Source: CAD feature listing. Evaluate the final solid. Frame: model axes, mm. Face numbers are marked on the shaded views. A direction names the side the tool comes from. Round coordinates to 2 decimals unless told otherwise and drop trailing zeros. Order: outer loops, then holes, each group sorted by start corner. A loop starts at its lowest first (then second) coordinate and runs counter-clockwise, first axis right, second up. Notation, with made-up numbers: (-26, 17) - (13, 17) arc R17 ccw to (13, 42) - close; hole circle Ø6 at (60, 69.5). An arc over 180 degrees is marked (long way). Return JSON: item names as keys, results as strings. Group by question number.
1) Section A-A, the plane z = -36.5. Return loops of the section in (x, y).
2) Ray query, line 1 (Y direction, x = 21, z = 45); line 2 (Y direction, x = 3, z = -17); line 3 (Z direction, x = 15, y = 56.5). Return the intervals inside material, ascending. Write a range as from..to.
3) Mould query, pull axis X, two halves, no side actions, for the marked faces 1, 2, 3 and 4. Classes: pulls with the +X half, pulls with the -X half, needs draft (parallel to the pull), parting line crosses it, or undercut.
4) Section C-C, the plane x = -23. Return loops of the section in (y, z), plus the area to 3 significant figures.
5) Contact query for flat-ended pins moving along their axis: P1, Ø9, axis at y = 33, z = 7, coming from the +X side; P2, Ø5.5, axis at y = 56.5, z = -3.5, coming from the +X side; P3, Ø8, axis at x = -34, y = 65.5, coming from the -Z side; P4, Ø6, axis at x = -4.5, y = 85, coming from the -Z side. Output: stop coordinate, or through.
6) Access query for the marked faces 5, 6, 7, 8 and 9. Directions: +Z, -Z, +X, -X, +Y, -Y. A direction counts if a zero-diameter tool reaches every point of the face in a straight line with its end or side. Return the directions, or none.
7) Section D-D, the plane z = 0. Return loops of the section in (x, y).
8) Section B-B, the plane x = 0. Return loops of the section in (y, z).
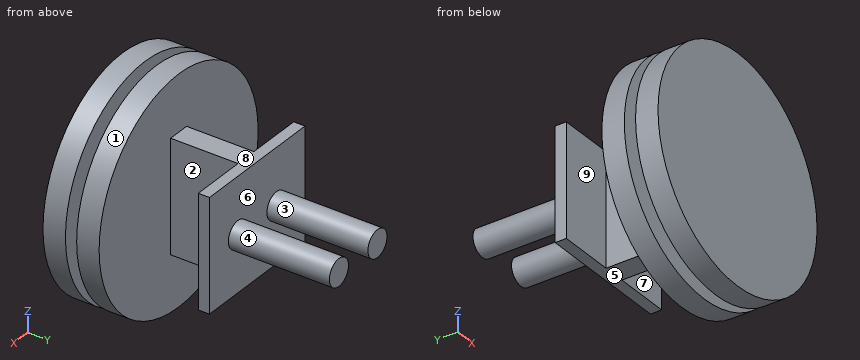
```python
from build123d import *

# Parameters (mm, degrees)
SKETCH_1_R      = 50
EXTRUDE_1_DEPTH = 10
SKETCH_2_R      = 10
EXTRUDE_2_DEPTH = 5
SKETCH_3_R      = 50
EXTRUDE_3_DEPTH = 10
SKETCH_4_W      = 10
SKETCH_4_H      = 50
EXTRUDE_4_DEPTH = 30
SKETCH_5_W      = 60
SKETCH_5_H      = 50
EXTRUDE_5_DEPTH = 5
SKETCH_6_R      = 6
EXTRUDE_6_DEPTH = 45


with BuildPart() as part:
    # 草图1 → 凸台-拉伸1 (new body)
    with BuildSketch(Plane(origin=(0, 0, 0), x_dir=(1, 0, 0), z_dir=(0, 1, 0))):
        with Locations(Location((0, 0, 0), (0, 0, 270))):
            Circle(SKETCH_1_R)
    extrude(amount=EXTRUDE_1_DEPTH)

    # 草图2 → 凸台-拉伸2 (add)
    with BuildSketch(Plane(origin=(0, 10, 0), x_dir=(1, 0, 0), z_dir=(0, 1, 0))):
        with Locations(Location((0, 0, 0), (0, 0, 270))):
            Circle(SKETCH_2_R)
    extrude(amount=EXTRUDE_2_DEPTH)

    # 草图3 → 凸台-拉伸3 (add)
    with BuildSketch(Plane(origin=(0, 15, 0), x_dir=(1, 0, 0), z_dir=(0, 1, 0))):
        with Locations(Location((0, 0, 0), (0, 0, 270))):
            Circle(SKETCH_3_R)
    extrude(amount=EXTRUDE_3_DEPTH)

    # 草图4 → 凸台-拉伸4 (add)
    with BuildSketch(Plane(origin=(0, 25, 0), x_dir=(1, 0, 0), z_dir=(0, 1, 0))):
        Rectangle(SKETCH_4_W, SKETCH_4_H)
    extrude(amount=EXTRUDE_4_DEPTH)

    # 草图5 → 凸台-拉伸5 (add)
    with BuildSketch(Plane(origin=(0, 55, 0), x_dir=(1, 0, 0), z_dir=(0, 1, 0))):
        Rectangle(SKETCH_5_W, SKETCH_5_H)
    extrude(amount=EXTRUDE_5_DEPTH)

    # 草图6 → 凸台-拉伸6 (add)
    with BuildSketch(Plane(origin=(0, 60, 0), x_dir=(1, 0, 0), z_dir=(0, 1, 0))):
        with Locations(Location((12.118185601, 0, 0), (0, 0, 90))):
            Circle(SKETCH_6_R)
        with Locations(Location((-12.118185601, 0, 0), (0, 0, 90))):
            Circle(SKETCH_6_R)
    extrude(amount=EXTRUDE_6_DEPTH)


solid = part.part
```
Geometry check:
{
 "1": {"outline": "(-34.17, 0) - (34.17, 0) - (34.17, 10) - (-34.17, 10) - close; (-34.17, 15) - (34.17, 15) - (34.17, 25) - (-34.17, 25) - close"},
 "2": {"line 1": "0..10, 15..25", "line 2": "0..10, 15..60", "line 3": "-25..25"},
 "3": {"face 1": "parting line crosses it", "face 2": "pulls with the +X half", "face 3": "undercut", "face 4": "undercut"},
 "4": {"outline": "(0, -44.4) - (10, -44.4) - (10, 44.4) - (0, 44.4) - close; (15, -44.4) - (25, -44.4) - (25, 44.4) - (15, 44.4) - close; (55, -25) - (60, -25) - (60, 25) - (55, 25) - close", "area": "2,030 mm2"},
 "5": {"P1": "x = 5", "P2": "x = 30", "P3": "through", "P4": "z = -3.83"},
 "6": {"face 5": "-Z, +X, -X, +Y", "face 6": "+Y", "face 7": "+Z, -Z, +X", "face 8": "+Z, +X, -X, +Y", "face 9": "+Z, -Z, -X"},
 "7": {"outline": "(-50, 0) - (50, 0) - (50, 10) - (10, 10) - (10, 15) - (50, 15) - (50, 25) - (5, 25) - (5, 55) - (30, 55) - (30, 60) - (18.12, 60) - (18.12, 105) - (6.12, 105) - (6.12, 60) - (-6.12, 60) - (-6.12, 105) - (-18.12, 105) - (-18.12, 60) - (-30, 60) - (-30, 55) - (-5, 55) - (-5, 25) - (-50, 25) - (-50, 15) - (-10, 15) - (-10, 10) - (-50, 10) - close"},
 "8": {"outline": "(0, -50) - (10, -50) - (10, -10) - (15, -10) - (15, -50) - (25, -50) - (25, -25) - (60, -25) - (60, 25) - (25, 25) - (25, 50) - (15, 50) - (15, 10) - (10, 10) - (10, 50) - (0, 50) - close"}
}
